from build123d import *

# Parameters (mm, degrees)
SKETCH1_R           = 7.5
BOSS_EXTRUDE1_DEPTH = 5
SKETCH3_R           = 10.5
BOSS_EXTRUDE2_DEPTH = 4
SKETCH4_R           = 8.25
CUT_EXTRUDE1_DEPTH  = 3
CHAMFER1_SIZE       = 0.5


with BuildPart() as part:
    # Sketch1 → Boss-Extrude1 (new body)
    with BuildSketch(Plane.XY):
        Circle(SKETCH1_R)
    extrude(amount=BOSS_EXTRUDE1_DEPTH)

    # Sketch3 → Boss-Extrude2 (add)
    with BuildSketch(Plane(origin=(0, 0, 0), x_dir=(-1, 0, 0), z_dir=(0, 0, -1))):
        Circle(SKETCH3_R)
    extrude(amount=BOSS_EXTRUDE2_DEPTH)

    # Sketch4 → Cut-Extrude1 (cut)
    with BuildSketch(Plane(origin=(0, 0, -4), x_dir=(-1, 0, 0), z_dir=(0, 0, -1))):
        Circle(SKETCH4_R)
    extrude(amount=-CUT_EXTRUDE1_DEPTH, mode=Mode.SUBTRACT)

    # Chamfer1
    chamfer1_edges = [part.edges().sort_by_distance(p)[0] for p in [
        (8.25, 0, -4),
    ]]
    chamfer(chamfer1_edges, length=CHAMFER1_SIZE)


solid = part.part
Work out the finished part from the listing and answer in its coordinate system (mm). A direction names the side the tool comes from. Give positions to 0.01 mm unless a question says otherwise; leave off trailing zeros. Order: outer loops, then holes, each group sorted by start corner. A loop starts at its lowest first (then second) coordinate and runs counter-clockwise, first axis right, second up. Notation, with made-up numbers: M 8,77 L 30,77 A36 ccw 30,112 Z; hole C 38.5,5 d11. An arc over 180 degrees is marked long. Return JSON: item names as keys, results as strings.
Q1. Find the intervals of material crossed by line 1 along Y through (x, z) = (0, -2.85); line 2 along Z through (x, y) = (1.25, 4.5); line 3 along Z through (x, y) = (-6, -7.5), in increasing order. Write a range as [from, to].
Answer below:
{"line 1": "y = [-10.5, -8.25], [8.25, 10.5]", "line 2": "z = [-1, 5]", "line 3": "z = [-4, 0]"}
Q2. Find section D-D, the plane z = 2.5. Write down the section's boundary in (x, y), and give its area (3 significant figures).
Answer below:
{"outline": "C 0,0 d15", "area": "177 mm^2"}
Q3. Find section A-A, the plane y = 0. Write down the section's boundary in (x, z).
Answer below:
{"outline": "M -10.5,-4 L -8.75,-4 L -8.25,-3.5 L -8.25,-1 L 8.25,-1 L 8.25,-3.5 L 8.75,-4 L 10.5,-4 L 10.5,0 L 7.5,0 L 7.5,5 L -7.5,5 L -7.5,0 L -10.5,0 Z"}
Q4. Which of the six approach directions +Z, -Z, +X, -X, +Y, -Y give full straight-line access (tool end or side, diameter ignored) to faces 4 (the face through (0, 0, 5)), 5 (the face through (-5, -7, 0)), 6 (the face through (-7.62, -3.16, -2.27))?
Answer below:
{"face 4": "+Z, +X, -X, +Y, -Y", "face 5": "+Z", "face 6": "-Z"}
Q5. Each of these flat-tipped pins is pushed along its axis until it touches: pin 1 (5 mm diameter, centred on x = 7.5, z = 3, fed in from -Y); pin 2 (1 mm diameter, centred on y = -5.5, z = -2.5, fed in from +X); pin 3 (4 mm diameter, centred on y = -6.5, z = 3.5, fed in from +X). Where does it stop, or does it pass through?
Answer below:
{"pin 1": "stops at y = -5.59", "pin 2": "stops at x = 9.23", "pin 3": "stops at x = 6"}
Q6. The mould has two halves that part along X. Classify faces 1 (the face through (0, 0, -1)), 2 (the face through (-7.493, 0.33, 2.465)), 3 (the face through (4, 8, -4)): pulls with the +X half, pulls with the -X half, needs draft (parallel to the pull), parting line crosses it, or undercut.
Answer below:
{"face 1": "undercut", "face 2": "parting line crosses it", "face 3": "needs draft"}
Q7. Find section C-C, the plane z = -1.5. Write down the section's boundary in (x, y), and give its area (3 significant figures).
Answer below:
{"outline": "C 0,0 d21; hole C 0,0 d16.5", "area": "133 mm^2"}
